CAD build for the part. Positions are in the model's coordinates, mm. A direction names the side the tool comes from. Round coordinates to 2 decimals unless told otherwise and drop trailing zeros. Order: outer loops, then holes, each group sorted by start corner. A loop starts at its lowest first (then second) coordinate and runs counter-clockwise, first axis right, second up.
Autodesk Inventor part; units mm, degrees
ref_plane "YZ Plane" through (0, 0, 0) normal (1, 0, 0) x (0, 1, 0)
ref_plane "XZ Plane" through (0, 0, 0) normal (0, 1, 0) x (-1, 0, 0)
ref_plane "XY Plane" through (0, 0, 0) normal (0, 0, 1) x (1, 0, 0)
sketch "Эскиз1" plane through (0, 0, 0) normal (0, 1, 0) x (-1, 0, 0)
  line L0 (85.25, 60) -> (-85.25, 60)
  line L1 (-85.25, 60) -> (-85.25, -60)
  line L2 (-85.25, -60) -> (85.25, -60)
  line L3 (85.25, -60) -> (85.25, 60)
  line L4 (85.25, 60) -> (-85.25, -60) construction
  line L5 (-85.25, 60) -> (85.25, -60) construction
  point P0 (0, 0)
  dimension "d0" = 170.5
  dimension "d1" = 120
extrude "Выдавливание1" add sketch "Эскиз1" along normal blind 4
sketch "Эскиз2" plane through (0, 4, 0) normal (0, 1, 0) x (1, 0, 0)
  circle A0 centre (-75.25, 8.7) radius 1.6
  circle A1 centre (75.25, 8.2) radius 1.6
  circle A2 centre (-75.25, -37.5) radius 1.6
  circle A3 centre (75.25, -38) radius 1.6
  point P0 (0, 0)
extrude "Выдавливание2" cut sketch "Эскиз2" against normal blind 4
chamfer "Фаска1" distance 8 angle 45 4 edges at (-85.25, 2, -60) (-85.25, 2, 60) (85.25, 2, -60) (85.25, 2, 60)
sketch "Эскиз3" plane through (0, 4, 0) normal (0, 1, 0) x (1, 0, 0)
  circle A0 centre (0, -50) radius 2.55
  circle A1 centre (0, -10) radius 2.55
  line L0 (-85.25, 52) -> (-85.25, -52)
  line L1 (-77.25, -60) -> (77.25, -60)
  point P0 (0, 0)
  dimension "d11" = 85.25
  dimension "d12" = 10
  dimension "d13" = 5.1
extrude "Выдавливание3" cut sketch "Эскиз3" against normal blind 10
sketch "Эскиз4" plane through (0, 4, 0) normal (0, 1, 0) x (1, 0, 0)
  circle A0 centre (0, -50) radius 2.55 construction
  line L0 (64, -38.5) -> (16, -38.5) construction
  line L1 (64, -36) -> (16, -36)
  line L2 (16, -41) -> (64, -41)
  arc A1 (64, -41) -> (64, -36) centre (64, -38.5) ccw
  arc A2 (16, -36) -> (16, -41) centre (16, -38.5) ccw
  line L3 (-77.25, -60) -> (77.25, -60) construction
  line L4 (0, -60) -> (0, 0) construction
  line L5 (50, 19) -> (-50, 19) construction
  line L6 (50, 22) -> (-50, 22)
  line L7 (-50, 16) -> (50, 16)
  arc A3 (50, 16) -> (50, 22) centre (50, 19) ccw
  arc A4 (-50, 22) -> (-50, 16) centre (-50, 19) ccw
  line L8 (0, 0) -> (0, 38) construction
  line L9 (-64, -38.5) -> (-16, -38.5) construction
  line L10 (-64, -36) -> (-16, -36)
  line L11 (-16, -41) -> (-64, -41)
  arc A5 (-64, -36) -> (-64, -41) centre (-64, -38.5) ccw
  arc A6 (-16, -41) -> (-16, -36) centre (-16, -38.5) ccw
  line L12 (77.25, -60) -> (-77.25, -60) construction
  point P0 (40, -38.5)
  point P1 (0, 19)
  point P2 (0, 19)
  point P3 (-40, -38.5)
  dimension "d14" = 24
  dimension "d15" = 5
  dimension "d16" = 16
  dimension "d17" = 50
  dimension "d18" = 6
  dimension "d21" = 16
extrude "Выдавливание4" cut sketch "Эскиз4" against normal blind 10
properties part number "фанера" material "Древесина (береза)"
1. Cut at C-C, the plane x = -8. Write the cut outline in (y, z).
2. Drill centre lines: line 1 (Z direction, x = -50, y = 3.6); line 2 (Z direction, x = -75.25, y = 1.45); line 3 (Z direction, x = 8.5, y = 1.1). Where is each one in solid material? Low to high.
3. Cut at D-D, the plane x = 46. Write the cut outline in (y, z), and give its area (3 significant figures).
4. Mould opens along Z. For faces 1 (the face through (81.31, 1.97, -55.94)), 2 (the face through (-66.5, 2, 38.4)), 3 (the face through (-0.33, 2.03, 47.47)), 4 (the face through (-1, 2, 60)) say: released by +Z, released by -Z, zero draft, split by the parting line, or undercut.
5. Tool access for faces 5 (the face through (1, 0, 1)), 6 (the face through (1, 2, -22)): list every direction of +Z, -Z, +X, -X, +Y, -Y with a clear straight run to the whole face (end or side of a thin tool).
6. Cut at A-A, the plane z = -19. Write the cut outline in (x, y).
7. Cut at B-B, the plane y = 1.55. Give the number of separate pieces and of enclosed holes in the cut face, and give its area (3 significant figures).
8. Pin check, flat tips, straight feed: P1, Ø8, axis at x = 0, z = 50, coming from the -Y side; P2, Ø3, axis at x = -75.25, z = 37.5, coming from the +Y side. Stop position of each tip, or through.
Outcome:
1. outline: (0, -60) - (4, -60) - (4, -22) - (0, -22) - close; (0, -16) - (4, -16) - (4, 60) - (0, 60) - close
2. line 1: z = -60 to -22, -16 to 36, 41 to 60
2. line 2: z = -60 to -10.3, -7.1 to 35.9, 39.1 to 60
2. line 3: z = -60 to -22, -16 to 60
3. outline: (0, -60) - (4, -60) - (4, -22) - (0, -22) - close; (0, -16) - (4, -16) - (4, 36) - (0, 36) - close; (0, 41) - (4, 41) - (4, 60) - (0, 60) - close
3. area: 436 mm2
4. face 1: released by -Z
4. face 2: undercut
4. face 3: undercut
4. face 4: released by +Z
5. face 5: +Z, -Z, +X, -X, -Y
5. face 6: +Y, -Y
6. outline: (-85.25, 0) - (-53, 0) - (-53, 4) - (-85.25, 4) - close; (53, 0) - (85.25, 0) - (85.25, 4) - (53, 4) - close
7. separate pieces: 1
7. enclosed holes: 9
7. area: 19,100 mm2
8. P1: stops at y = 0
8. P2: passes through
